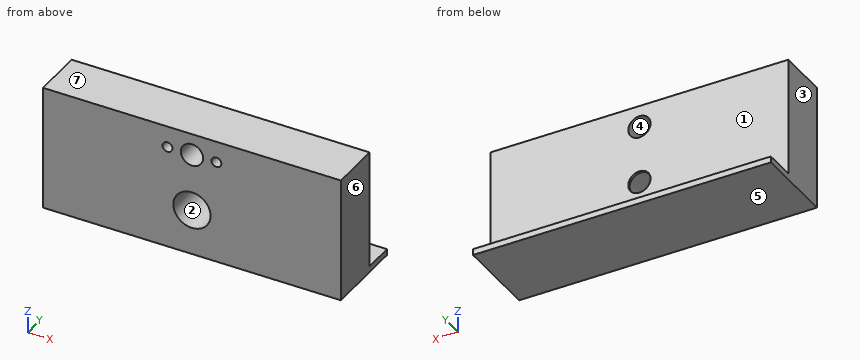
Autodesk Inventor part; units mm, degrees
ref_plane "YZ Plane" through (0, 0, 0) normal (1, 0, 0) x (0, 1, 0)
ref_plane "XZ Plane" through (0, 0, 0) normal (0, 1, 0) x (-1, 0, 0)
ref_plane "XY Plane" through (0, 0, 0) normal (0, 0, 1) x (1, 0, 0)
sketch "Sketch1" plane through (0, 0, 0) normal (0, 1, 0) x (-1, 0, 0)
  line L0 (0, 0) -> (30.48, 0)
  line L1 (30.48, 0) -> (-30.48, 0)
  line L2 (-30.48, 0) -> (-30.48, -15.748)
  line L3 (-30.48, -15.748) -> (30.48, -15.748)
  line L4 (30.48, -15.748) -> (30.48, 0)
  line L5 (30.48, -15.748) -> (30.48, -15.494)
  line L6 (30.48, -15.494) -> (-30.48, -15.494)
  line L7 (0, 0) -> (0, -7.366)
  circle A0 centre (0, -7.366) radius 2.286
  line L8 (30.48, 0) -> (30.48, 8.89)
  line L9 (30.48, 8.89) -> (-30.48, 8.89)
  line L10 (-30.48, 8.89) -> (-30.48, 0)
  line L11 (30.48, 0) -> (-30.48, 0)
  line L12 (0, 0) -> (0, 4.445)
  circle A1 centre (0, 4.445) radius 2.286
  line L13 (30.48, -15.748) -> (-30.48, -15.748)
  line L14 (-30.48, -15.748) -> (-30.48, -16.7568)
  line L15 (-30.48, -16.7568) -> (30.48, -16.7568)
  line L16 (30.48, -16.7568) -> (30.48, -15.748)
  dimension "d0" = 30.48
  dimension "d1" = 60.96
  dimension "d2" = 15.748
  dimension "d3" = 0.254
  dimension "d4" = 7.366
  dimension "d5" = 4.572
  dimension "d14" = 8.89
  dimension "d15" = 4.572
extrude "Extrusion1" add sketch "Sketch1" along normal blind 10.414 contours L0 L4 L6 L2 L1
extrude "Extrusion2" add sketch "Sketch1" along normal blind 16.764 contours L4 L3 L2 L6 | L16 L15 L14 L3
sketch "Sketch2" plane through (0, 0, 0) normal (0, -1, 0) x (1, 0, 0)
  line L0 (0, 0) -> (0, -7.366)
  circle A0 centre (0, -7.366) radius 3.81
  dimension "d10" = 7.366
  dimension "d11" = 7.62
extrude "Extrusion3" cut sketch "Sketch2" against normal blind 9.906
extrude "Extrusion4" add sketch "Sketch1" along normal blind 10.414 contours L1 L10 L9 L8 L0
sketch "Sketch3" plane through (0, 0, 0) normal (0, -1, 0) x (1, 0, 0)
  line L0 (0, 4.5142) -> (5.0038, 4.5142)
  line L1 (0, 4.5142) -> (-5.0038, 4.5142)
  circle A0 centre (5.0038, 4.5142) radius 1.0109
  circle A1 centre (-5.0038, 4.5142) radius 1.0109
  point P0 (0, 0)
  dimension "d18" = 5.0038
  dimension "d19" = 5.0038
  dimension "d20" = 2.0218
  dimension "d21" = 2.0218
extrude "Extrusion5" cut sketch "Sketch3" against normal blind 4.445
properties part number "RotationMounttoPolarisPinAdapter"
Build history of the part. All positions in model axes, mm. Face numbers are marked on the shaded views. A direction names the side the tool comes from. Give positions to 0.01 mm unless a question says otherwise; leave off trailing zeros. Order: outer loops, then holes, each group sorted by start corner. A loop starts at its lowest first (then second) coordinate and runs counter-clockwise, first axis right, second up. Notation, with made-up numbers: M -20,-35 L 15,-35 A17 cw 15,-13 Z; hole C -4.75,-5 d4. An arc over 180 degrees is marked long. Use one line per item in the form item = value.
1) Saw through at D-D (z = -12.25). Give the cut face in (x, y).
Calculated:
outline = M -30.48,0 L 30.48,0 L 30.48,10.41 L -30.48,10.41 Z
2) Two-plate mould, pull along Z, no slides. Class the marked faces 4, 5, 6 and 7: released by +Z, released by -Z, zero draft, split by the parting line, or undercut.
Calculated:
face_4 = undercut
face_5 = released by -Z
face_6 = zero draft
face_7 = released by +Z
3) Saw through at B-B (z = -6.25). Give the cut face in (x, y), plus the area to 3 significant figures.
Calculated:
outline = M -30.48,0 L -3.64,0 L -3.64,9.91 L -2,9.91 L -2,10.41 L -30.48,10.41 Z; M 2,9.91 L 3.64,9.91 L 3.64,0 L 30.48,0 L 30.48,10.41 L 2,10.41 Z
area = 561 mm2
4) Saw through at C-C (x = -18). Give the cut face in (y, z), plus the area to 3 significant figures.
Calculated:
outline = M 0,-16.76 L 16.76,-16.76 L 16.76,-15.49 L 10.41,-15.49 L 10.41,8.89 L 0,8.89 Z
area = 275 mm2
5) Drop flat-ended pins along their axis: pin 1 (1 mm diameter, centred on x = 6.5, y = 11, fed in from +Z); pin 2 (2 mm diameter, centred on x = -5.5, z = 5, fed in from -Y); pin 3 (1.6 mm diameter, centred on x = -5, z = 4.51, fed in from +Y); pin 4 (7 mm diameter, centred on x = 0, z = -7.366, fed in from -Y). Give the stop position or say it passes through.
Calculated:
pin_1 = -15.49
pin_2 = 0
pin_3 = 10.41
pin_4 = 9.91
6) Saw through at A-A (x = 0). Give the cut face in (y, z), plus the area to 3 significant figures.
Calculated:
outline = M 0,-16.76 L 16.76,-16.76 L 16.76,-15.49 L 10.41,-15.49 L 10.41,-9.65 L 9.91,-9.65 L 9.91,-11.18 L 0,-11.18 Z; M 0,-3.56 L 9.91,-3.56 L 9.91,-5.08 L 10.41,-5.08 L 10.41,2.16 L 0,2.16 Z; M 0,6.73 L 10.41,6.73 L 10.41,8.89 L 0,8.89 Z
area = 150 mm2
7) Probe probe 1 along Z at (x, y) = (0, 2.5); probe 2 along X at (y, z) = (5, -7.25); probe 3 along Z at (x, y) = (0, 10.35). List the from-to ranges inside material, lowest first.
Calculated:
probe_1 = -16.76 to -11.18, -3.56 to 2.16, 6.73 to 8.89
probe_2 = -30.48 to -3.81, 3.81 to 30.48
probe_3 = -16.76 to -9.65, -5.08 to 2.16, 6.73 to 8.89
8) Tool access for the marked faces 1, 2 and 3: list every direction of +Z, -Z, +X, -X, +Y, -Y with a clear straight run to the whole face (end or side of a thin tool).
Calculated:
face_1 = +Z, +X, -X, +Y
face_2 = -Y
face_3 = +Z, -Z, -X, +Y, -Y
